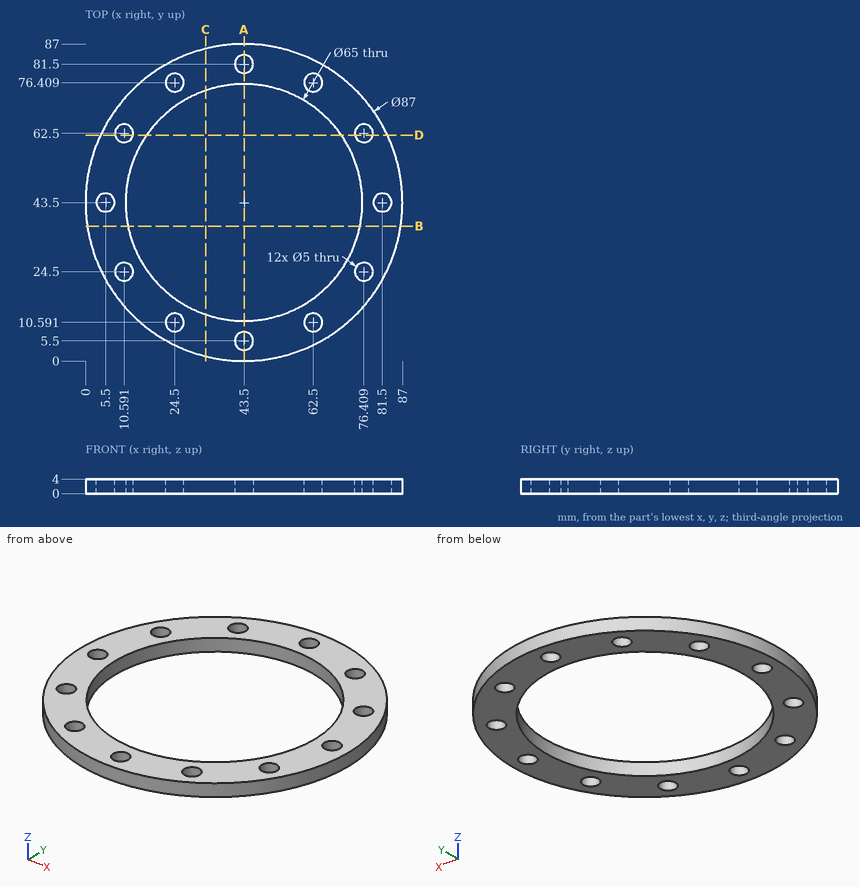
Part print with two shaded views. Sizes in mm from the minimum x, y, z corner. Round coordinates to 2 decimals unless told otherwise and drop trailing zeros. Loops run counter-clockwise (first coordinate to the right, second up) from the corner with the lowest first, then second, coordinate; pieces in that order, holes last.
1. Slice it at D-D (y = 62). Give the cut face in (x, z).
Solutions:
outline: (4.13, 0) - (8.14, 0) - (8.14, 4) - (4.13, 4) - close; (13.04, 0) - (16.78, 0) - (16.78, 4) - (13.04, 4) - close; (70.22, 0) - (73.96, 0) - (73.96, 4) - (70.22, 4) - close; (78.86, 0) - (82.87, 0) - (82.87, 4) - (78.86, 4) - close
2. Slice it at B-B (y = 37). Give the cut face in (x, z).
Solutions:
outline: (0.49, 0) - (11.66, 0) - (11.66, 4) - (0.49, 4) - close; (75.34, 0) - (86.51, 0) - (86.51, 4) - (75.34, 4) - close
3. Slice it at C-C (x = 33). Give the cut face in (y, z).
Solutions:
outline: (1.29, 0) - (12.74, 0) - (12.74, 4) - (1.29, 4) - close; (74.26, 0) - (85.71, 0) - (85.71, 4) - (74.26, 4) - close
4. Slice it at A-A (x = 43.5). Give the cut face in (y, z), and give its area (3 significant figures).
Solutions:
outline: (0, 0) - (3, 0) - (3, 4) - (0, 4) - close; (8, 0) - (11, 0) - (11, 4) - (8, 4) - close; (76, 0) - (79, 0) - (79, 4) - (76, 4) - close; (84, 0) - (87, 0) - (87, 4) - (84, 4) - close
area: 48.0 mm2
5. Drill centre lines: line 1 along X through (y, z) = (77, 3.65); line 2 along X through (y, z) = (77.5, 2.45); line 3 along Y through (x, z) = (45, 2.2). Where is each one in solid material? Low to high.
Solutions:
line 1: x = 15.75 to 22.07, 26.93 to 60.07, 64.93 to 71.25
line 2: x = 16.37 to 22.25, 26.75 to 60.25, 64.75 to 70.63
line 3: y = 0.03 to 3.5, 7.5 to 11.03, 75.97 to 79.5, 83.5 to 86.97
6. Flat gauge pins, fed straight in: pin 1 (6.5 mm diameter, centred on x = 76.41, y = 62.5, fed in from -Z); pin 2 (1 mm diameter, centred on y = 9, z = 2, fed in from +X); pin 3 (1 mm diameter, centred on x = 67, z = 2, fed in from +Y). Where does each tip first touch, or does it go through?
Solutions:
pin 1: stops at z = 0
pin 2: stops at x = 70.63
pin 3: stops at y = 80.42
